```python
from build123d import *

# Parameters (mm, degrees)
CADVIEW_START                   = -9.527864724
CADVIEW_RADIAL_HOLE_PROFILE_1_R = 2.48285337
CADVIEW_RADIAL_HOLE_1_DEPTH     = 1.211153441
CADVIEW_START_2                 = 9.883993552
CADVIEW_RADIAL_HOLE_PROFILE_3_R = 1.487902792
CADVIEW_RADIAL_HOLE_3_DEPTH     = 1.33410702
CADVIEW_START_3                 = 9.529411148
CADVIEW_RADIAL_HOLE_PROFILE_2_R = 2.482933282
CADVIEW_RADIAL_HOLE_2_DEPTH     = 1.211645438
CADVIEW_START_4                 = -9.883175541
CADVIEW_RADIAL_HOLE_PROFILE_4_R = 1.487684902
CADVIEW_RADIAL_HOLE_4_DEPTH     = 1.33397788


with BuildPart() as part:
    # CADView Revolve Profile → CADView Core Revolve (revolve)
    with BuildSketch(Plane.XY, mode=Mode.PRIVATE) as cadview_core_revolve_sk:
        Polygon((11.191399791, 0), (11.191653126, 9.441445801), (10.600473645, 10.104003401), (10.21110818, 10.766561001), (9.973962294, 11.429118601), (9.844267199, 12.422955001), (9.96776039, 13.416791401), (10.199820897, 14.079349001), (10.58298579, 14.741906601), (11.17653503, 15.404464201), (11.191453753, 16.729579401), (11.044622402, 17.060858201), (10.490300644, 17.723415801), (10.142815737, 18.385973401), (9.936295224, 19.048531001), (9.847392508, 20.042367401), (9.928006815, 20.704925001), (10.127236671, 21.367482602), (10.464744973, 22.030040202), (11.006241128, 22.692597802), (11.19151131, 23.023876602), (11.191468831, 29.649452602), (6.217451578, 29.980731402), (6.217426324, 31.802764802), (3.357168025, 31.802764802), (3.357285746, 26.005385802), (8.704312973, 25.674107002), (8.704166835, 0), align=None)
    revolve(cadview_core_revolve_sk.sketch.rotate(Axis((0, 0, 0), (0, 1, 0)), 90), axis=Axis((0, 0, 0), (0, 1, 0)))

    # CADView Radial Hole Profile 1 → CADView Radial Hole 1 (cut, symmetric)
    with BuildSketch(Plane.XY.offset(CADVIEW_START)):
        with Locations(Location((7.8903e-05, 19.896357505, 0), (0, 0, 3.371355006))):
            Circle(CADVIEW_RADIAL_HOLE_PROFILE_1_R)
    extrude(amount=CADVIEW_RADIAL_HOLE_1_DEPTH, both=True, mode=Mode.SUBTRACT)

    # CADView Radial Hole Profile 3 → CADView Radial Hole 3 (cut, symmetric)
    with BuildSketch(Plane(origin=(0, 0, 0), x_dir=(0, 0, -1), z_dir=(1, 0, 0)).offset(CADVIEW_START_2)):
        with Locations(Location((0.000122905, 4.974426113, 0), (0, 0, 315.785142597))):
            Circle(CADVIEW_RADIAL_HOLE_PROFILE_3_R)
    extrude(amount=CADVIEW_RADIAL_HOLE_3_DEPTH, both=True, mode=Mode.SUBTRACT)

    # CADView Radial Hole Profile 2 → CADView Radial Hole 2 (cut, symmetric)
    with BuildSketch(Plane.XY.offset(CADVIEW_START_3)):
        with Locations(Location((0.000277866, 12.43536503, 0), (0, 0, 359.713626975))):
            Circle(CADVIEW_RADIAL_HOLE_PROFILE_2_R)
    extrude(amount=CADVIEW_RADIAL_HOLE_2_DEPTH, both=True, mode=Mode.SUBTRACT)

    # CADView Radial Hole Profile 4 → CADView Radial Hole 4 (cut, symmetric)
    with BuildSketch(Plane(origin=(0, 0, 0), x_dir=(0, 0, -1), z_dir=(1, 0, 0)).offset(CADVIEW_START_4)):
        with Locations(Location((2.8248e-05, 4.974003332, 0), (0, 0, 315.785395623))):
            Circle(CADVIEW_RADIAL_HOLE_PROFILE_4_R)
    extrude(amount=CADVIEW_RADIAL_HOLE_4_DEPTH, both=True, mode=Mode.SUBTRACT)


solid = part.part
```
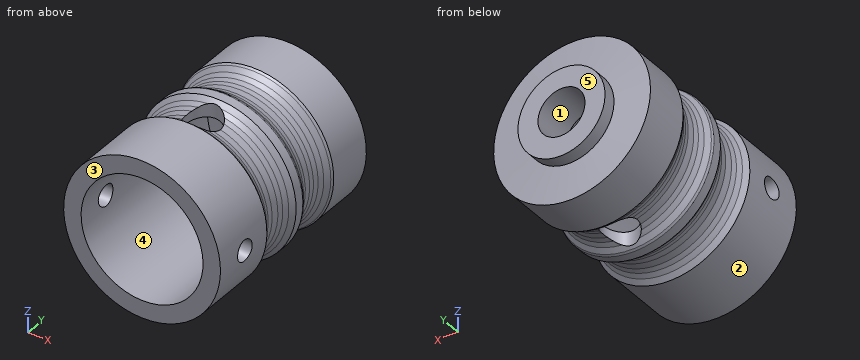
Geometry: final body of the model. Coordinates: model frame, mm. Face numbers are marked on the shaded views. A direction names the side the tool comes from. Round coordinates to 2 decimals unless told otherwise and drop trailing zeros. Loops run counter-clockwise (first coordinate to the right, second up) from the corner with the lowest first, then second, coordinate; pieces in that order, holes last. Notation, with made-up numbers: (53.5, -1.75) -> (71.5, -1.75) arc R4 ccw to (71.5, 5.25) -> close; hole circle Ø6 at (-28, 4.25). An arc over 180 degrees is marked (long way). Use one line per item in the form item = value. Start each with the question number.
1) Line query: L1, parallel to Y at x = 10, z = -3.5; L2, parallel to Z at x = -5.75, y = 18; L3, parallel to Z at x = 2.25, y = 28. Output: solid intervals per line, ascending.
2) Section A-A on y = 5.5. Output: boundary loops of the cut face in (x, z), then the cut area to 3 significant figures.
3) Section B-B on z = 0. Give the number of separate pieces and of enclosed holes in the cut face, then the cut area to 3 significant figures.
4) Access query for the marked faces 4 and 5. Directions: +Z, -Z, +X, -X, +Y, -Y. A direction counts if a zero-diameter tool reaches every point of the face in a straight line with its end or side. Return the directions, or none.
5) First-contact query: P1, Ø1.5, axis at x = -5.5, y = 26.5, coming from the -Z side; P2, Ø5, axis at y = 22.5, z = 3.5, coming from the +X side; P3, Ø10, axis at y = 28.5, z = 5.5, coming from the -X side. Flat tips, straight axial feed; report the tip coordinate or a pass-through.
6) Draft query along Z for the marked faces 1, 2 and 3. Return one class per face: released by +Z, released by -Z, zero draft, split by the parting line, or undercut.
Response:
q1.L1 = 0 to 10.11, 14.76 to 17.6, 22.19 to 29.69
q1.L2 = -8.6 to -6.53, 6.53 to 8.6
q1.L3 = -10.96 to -2.49, 2.49 to 10.96
q2.outline = (-11.1, -1.39) arc R11.19 ccw to (11.1, -1.39) -> (8.59, -1.39) arc R8.7 cw to (-8.59, -1.39) -> close; (-11.1, 1.39) -> (-8.59, 1.39) arc R8.7 cw to (8.59, 1.39) -> (11.1, 1.39) arc R11.19 ccw to start
q2.area = 142 mm^2
q3.separate_pieces = 4
q3.enclosed_holes = 0
q3.area = 165 mm^2
q4.face_4 = -Y
q4.face_5 = +Z, -Z, +X, -X, +Y
q5.P1 = -10.13
q5.P2 = 11.14
q5.P3 = -11.18
q6.face_1 = undercut
q6.face_2 = split by the parting line
q6.face_3 = zero draft
